from build123d import *

# Parameters (mm, degrees)
SKETCH_W     = 145
SKETCH_H     = 50
SKETCH_R     = 8
SKETCH_W_2   = 73
SKETCH_H_2   = 25
PAD_DEPTH    = 2
PAD001_DEPTH = 5


with BuildPart() as part:
    # Sketch → Pad (new body)
    with BuildSketch(Plane.XY):
        with Locations((72.5, 25)):
            Rectangle(SKETCH_W, SKETCH_H)
        with Locations((15, 13.5)):
            Circle(SKETCH_R, mode=Mode.SUBTRACT)
        with Locations((15, 36.5)):
            Circle(SKETCH_R, mode=Mode.SUBTRACT)
        with Locations((130, 13.5)):
            Circle(SKETCH_R, mode=Mode.SUBTRACT)
        with Locations((130, 36.5)):
            Circle(SKETCH_R, mode=Mode.SUBTRACT)
        with Locations((72.5, 25)):
            Rectangle(SKETCH_W_2, SKETCH_H_2, mode=Mode.SUBTRACT)
    extrude(amount=PAD_DEPTH)

    # Sketch001 (on Face14 of Pad) → Pad001 (join)
    with BuildSketch(Plane.XY.offset(2)):
        Polygon((36, 12.5), (109, 12.5), (114, 12.5), (114, 7.5), (109, 7.5), (109, 11.5), (31, 11.5), (31, 42.5), (109, 42.5), (114, 42.5), (114, 37.5), (109, 37.5), (36, 37.5), align=None)
    extrude(amount=PAD001_DEPTH)


solid = part.part
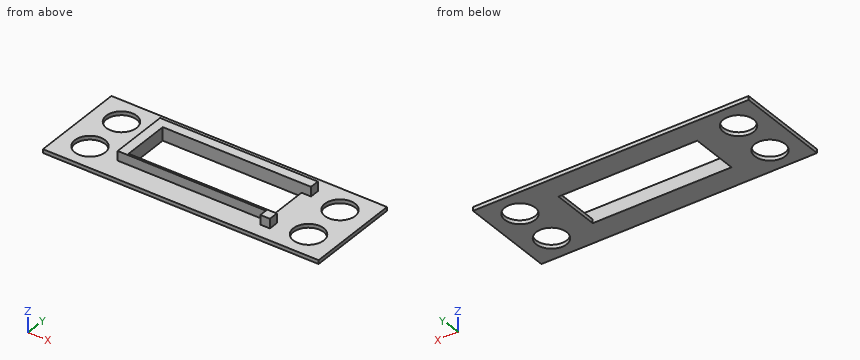
CAD build for the part. Positions are in the model's coordinates, mm. Round coordinates to 2 decimals unless told otherwise and drop trailing zeros. Order: outer loops, then holes, each group sorted by start corner. A loop starts at its lowest first (then second) coordinate and runs counter-clockwise, first axis right, second up. Notation, with made-up numbers: (19, 48.5) - (36, 48.5) arc R18 ccw to (36, 79.5) - close; hole circle Ø1 at (-17.75, -28). An arc over 180 degrees is marked (long way). Return JSON: item names as keys, results as strings.
(1) Wall check: probe 1 along Y at (x, z) = (130, 1.5); probe 2 along Y at (x, z) = (40.5, 2.5); probe 3 along Y at (x, z) = (68, 1). Give the ranges that are in metal, low to high. Write a range as from..to.
Answer key:
{"probe 1": "y = 0..5.5, 21.5..28.5, 44.5..50", "probe 2": "y = 11.5..12.5, 37.5..42.5", "probe 3": "y = 0..12.5, 37.5..50"}
(2) Cut at D-D (y = 46.5). Give the cut face in (x, z), then the cut area to 3 significant figures.
Answer key:
{"outline": "(0, 0) - (145, 0) - (145, 2) - (0, 2) - close", "area": "290 mm^2"}
(3) Cut at B-B (y = 10). Give the cut face in (x, z), then the cut area to 3 significant figures.
Answer key:
{"outline": "(0, 0) - (7.81, 0) - (7.81, 2) - (0, 2) - close; (22.19, 0) - (122.81, 0) - (122.81, 2) - (114, 2) - (114, 7) - (109, 7) - (109, 2) - (22.19, 2) - close; (137.19, 0) - (145, 0) - (145, 2) - (137.19, 2) - close", "area": "257 mm^2"}
(4) Cut at A-A (x = 17.5). Give the cut face in (y, z), then the cut area to 3 significant figures.
Answer key:
{"outline": "(0, 0) - (5.9, 0) - (5.9, 2) - (0, 2) - close; (21.1, 0) - (28.9, 0) - (28.9, 2) - (21.1, 2) - close; (44.1, 0) - (50, 0) - (50, 2) - (44.1, 2) - close", "area": "39.2 mm^2"}
(5) Cut at C-C (z = 5.5). Give the cut face in (x, y).
Answer key:
{"outline": "(31, 11.5) - (109, 11.5) - (109, 7.5) - (114, 7.5) - (114, 12.5) - (36, 12.5) - (36, 37.5) - (114, 37.5) - (114, 42.5) - (31, 42.5) - close"}
(6) Pin check, flat tips, straight feed: pin 1 Ø14.5 at (x, y) = (130, 36.5) entering from +Z; pin 2 Ø1.5 at (x, z) = (70, 4) entering from -Y; pin 3 Ø2.5 at (y, z) = (10, 3.5) entering from +X; pin 4 Ø2.5 at (y, z) = (32.5, 5.5) entering from -X. Stop position of each tip, or through.
Answer key:
{"pin 1": "passes through", "pin 2": "stops at y = 11.5", "pin 3": "stops at x = 114", "pin 4": "stops at x = 31"}
